CAD build for the part. Positions are in the model's coordinates, mm. A direction names the side the tool comes from. Coordinates: 2 decimals unless noted, no trailing zeros. Write each loop counter-clockwise with the first axis right and the second up, starting at its lowest first coordinate (ties: lowest second). Pieces come first, ordered by that corner, then holes. Notation, with made-up numbers: (0, 72.5) - (28, 72.5) arc R11 cw to (28, 77.5) - close; hole circle Ø1 at (-20, 80.5). An arc over 180 degrees is marked (long way). One line per question, with ' | ' between items. Start each with the question number.
1. Band-saw the part on D-D, the plane y = 10.5. Write the cut outline in (x, z).
2. Which spindle directions (+Z, -Z, +X, -X, +Y, -Y) get a long thin tool onto all of the face, cutting with end or side? Do faces 5 (the flat face through (32, 6, 1)), 6 (the flat face through (27, -13, 1)), 7 (the flat face through (18.2, 59.7, 1.2)), 8 (the flat face through (5, 8.85, 9)), 9 (the flat face through (4.56, 22.14, 1.01)). Say none if no direction does.
3. Probe line 1 (Y direction, x = 30, z = 6); line 2 (Y direction, x = 5.5, z = 11.75); line 3 (X direction, y = 8, z = 17). List the from-to ranges inside material, lowest first.
4. Band-saw the part on B-B, the plane x = 37. Write the cut outline in (y, z).
5. Two-plate mould, pull along Y, no slides. Class faces 1 (the flat face through (29, -8.65, 9)), 2 (the flat face through (30.5, 48.3, 16.5)), 3 (the flat face through (7, 0, 9)), 4 (the flat face through (0.7, 29.2, 9.1)): +Y half, -Y half, draft (parallel to the pull), parting line (faces both ways), or undercut.
6. Flat gauge pins, fed straight in: P1, Ø4.5, axis at y = 50, z = 5, coming from the +X side; P2, Ø1.2, axis at x = 29, z = 5.5, coming from the +Y side; P3, Ø0.9, axis at y = 59, z = 7, coming from the -X side; P4, Ø12, axis at x = 34, y = 28.5, coming from the +Z side. Where does each tip first touch, or does it go through?
7. Band-saw the part on C-C, the plane y = 39. Write the cut outline in (x, z), then the cut area to 3 significant figures.
8. Band-saw the part on A-A, the plane y = -4.5. Write the cut outline in (x, z).
Autodesk Fusion 360 part; units mm, degrees
sketch "Sketch1" plane through (0, 0, 0) normal (0, 0, 1) x (1, 0, 0)
  line L0 (0, 0) -> (0, 8.85)
  line L1 (0, 8.85) -> (9, 8.85)
  line L2 (9, 8.85) -> (9, 21.15)
  line L3 (9, 21.15) -> (0, 21.15)
  line L4 (0, 21.15) -> (0, 30)
  line L5 (0, 0) -> (12, 0)
  line L6 (26, 30) -> (31.5, 35.5)
  line L7 (31.5, 35.5) -> (31.5, 63.5)
  line L8 (0, 30) -> (12, 30)
  line L9 (21.5, 47.35) -> (21.5, 55.65) construction
  line L10 (17, 63.5) -> (31.5, 63.5)
  arc A0 (21.5, 47.35) -> (21.5, 55.65) centre (21.5, 51.5) ccw
  line L11 (21.5, 47.35) -> (17, 47.35)
  line L12 (17, 47.35) -> (12, 30)
  line L13 (21.5, 55.65) -> (17, 55.65)
  line L14 (17, 55.65) -> (17, 63.5)
  line L15 (30, -8.65) -> (30, -0.35) construction
  line L16 (30, -0.35) -> (25.5, -0.35)
  line L17 (30, -8.65) -> (25.5, -8.65)
  arc A1 (30, -8.65) -> (30, -0.35) centre (30, -4.5) ccw
  line L18 (12, 0) -> (25.5, -0.35)
  line L19 (25.5, -8.65) -> (25.5, -16.5)
  line L20 (25.5, -16.5) -> (40, -16.5)
  line L21 (40, -16.5) -> (40, 7.5)
  line L22 (40, 7.5) -> (26, 7.5)
  line L23 (26, 7.5) -> (26, 30)
  dimension "d3" = 9
  dimension "d4" = 12.3
  dimension "d6" = 30
  dimension "d7" = 21.5
  dimension "d8" = 51.5
  dimension "d10" = 8.3
  dimension "d13" = 17
  dimension "d14" = 10
  dimension "d15" = 12
  dimension "d20" = 12
  dimension "d22" = 12
  dimension "d25" = 4.5
  dimension "d26" = 30
  dimension "d27" = 12
  dimension "d28" = 10
  dimension "d29" = 12
  dimension "d32" = 26
  dimension "d33" = 45
extrude "Extrude1" add sketch "Sketch1" along normal blind 18
chamfer "Chamfer1" distance 2 distance2 3 13 edges at (31.5, 49.5, 18) (28.75, 32.75, 18) (28.75, 32.75, 0) (17, 63.5, 9) (14.5, 38.675, 18) (14.5, 38.675, 0) (17, 59.575, 18) (17, 59.575, 0) (33, 7.5, 18) (40, -4.5, 18) (33, 7.5, 0) (25.5, -12.575, 18) (25.5, -12.575, 0) measured on face at (20.3333, 19.55, 18) measured on face at (20.3333, 19.55, 18) measured on face at (27.8333, 31.8333, 6) measured on face at (21.8333, 63.5, 6) measured on face at (20.3333, 19.55, 18) measured on face at (15.3333, 41.5667, 6) measured on face at (20.3333, 19.55, 18) measured on face at (20.3333, 19.55, 0) measured on face at (20.3333, 19.55, 18) measured on face at (20.3333, 19.55, 18) measured on face at (35.3333, 7.5, 12) measured on face at (20.3333, 19.55, 18) measured on face at (25.5, -13.8833, 12)
chamfer "Chamfer2" distance 4 angle 45 3 edges at (31.5, 63.5, 7.5) (40, -16.5, 7.5) (40, 7.5, 8.5)
chamfer "Chamfer3" distance 2 angle 45 3 edges at (17, 55.65, 9) (17, 47.35, 8.5) (25.5, -8.65, 8.5)
chamfer "Chamfer4" distance 1.5 angle 45 4 edges at (0, 21.15, 9) (0, 8.85, 9) (0, 30, 9) (0, 0, 9)
chamfer "Chamfer5" distance 2 angle 45 4 edges at (5.25, 21.15, 18) (5.25, 8.85, 18) (5.25, 21.15, 0) (5.25, 8.85, 0)
chamfer "Chamfer7" distance 1 angle 45 12 edges at (25.65, 51.5, 0) (20.25, 55.65, 0) (20.811, 47.35, 0) (25.65, 51.5, 18) (20.2907, 47.35, 18) (20.25, 55.65, 18) (34.15, -4.5, 18) (28.75, -8.65, 18) (27.75, -0.35, 18) (34.15, -4.5, 0) (27.75, -0.35, 0) (29.25, -8.65, 0)
Filled in:
1) outline: (9, 0) - (26, 0) - (26, 18) - (9, 18) - close
2) face 5: -Z, +X | face 6: -Z, -X, -Y | face 7: -Z, -X, +Y | face 8: +Z, -Z, -X | face 9: -Z, -X
3) line 1: y = -16.5 to -8.65, -0.35 to 7.5, 34 to 61 | line 2: y = 0 to 8.85, 21.15 to 30 | line 3: x = 9 to 26
4) outline: (-15.5, 0) - (4.5, 0) - (6.5, 1.33) - (6.5, 16.5) - (5.5, 18) - (-15.5, 18) - close
5) face 1: undercut | face 2: draft | face 3: -Y half | face 4: +Y half
6) P1: stops at x = 31.5 | P2: stops at y = 62.6 | P3: stops at x = 17 | P4: passes through
7) outline: (14.59, 2) - (17.72, 0) - (30.76, 0) - (31.5, 0.35) - (31.5, 15) - (29.5, 18) - (16.68, 18) - (14.59, 15) - close | area: 295 mm²
8) outline: (34.15, 1) - (35.15, 0) - (40, 0) - (40, 15) - (38, 18) - (35.15, 18) - (34.15, 17) - close
